```python
from build123d import *

# Parameters (mm, degrees)
CHAMFER1_SIZE = 0.45


with BuildPart() as part:
    # Sketch1 → Revolve1 (revolve)
    with BuildSketch(Plane.XY):
        Polygon((3.25, 0), (3.25, 30.33), (9.44, 30.33), (9.44, 26.03), (11.225, 26.03), (11.225, 24.03), (10.225, 24.03), (10.225, 23.03), (11.225, 23.03), (11.225, 20.53), (12, 20.53), (12, 14.93), (10, 14.93), (10, 12.7), (9.46, 12.7), (9.46, 0), align=None)
    revolve(axis=Axis((0, 0, 0), (0, 1, 0)))

    # Chamfer1
    chamfer1_edges = [part.edges().sort_by_distance(p)[0] for p in [
        (-9.46, 0, 0),
        (-10, 14.93, 0),
        (-3.25, 0, 0),
    ]]
    chamfer(chamfer1_edges, length=CHAMFER1_SIZE)


solid = part.part
```
Here's how the part is built. I have some questions about the finished solid (model axes, mm). A direction names the side the tool comes from. Round coordinates to 2 decimals unless told otherwise and drop trailing zeros. Loops run counter-clockwise (first coordinate to the right, second up) from the corner with the lowest first, then second, coordinate; pieces in that order, holes last.
1. If I drill on probe 1 along X at (y, z) = (23.75, 0) (3 decimals); probe 2 along Z at (x, y) = (0, 13); probe 3 along Y at (x, z) = (-10.5, -2.5), over which ranges is the centre line in solid material (lowest first)?
Answers:
probe 1: x = -10.225 to -3.25, 3.25 to 10.225
probe 2: z = -10 to -3.25, 3.25 to 10
probe 3: y = 14.93 to 23.03, 24.03 to 26.03
2. Suppose I cut it at B-B, the plane y = 24.5. Please give me the cut outline in (x, z) (3 decimals).
Answers:
outline: circle Ø22.45 at (0, 0); hole circle Ø6.5 at (0, 0)
3. Will these pins go through, and if not, where does the flat tip stop? pin 1 (2 mm diameter, centred on x = 5, y = 9.5, fed in from -Z); pin 2 (1 mm diameter, centred on y = 14, z = -2, fed in from +X); pin 3 (1 mm diameter, centred on x = -9.5, z = -7, fed in from -Y).
Answers:
pin 1: stops at z = -8.57
pin 2: stops at x = 9.89
pin 3: stops at y = 14.93
4. Suppose I cut it at A-A, the plane y = 7.5. Please give me the cut outline in (x, z).
Answers:
outline: circle Ø18.92 at (0, 0); hole circle Ø6.5 at (0, 0)
5. For faces 1 (the face through (-11.99, 17.69, -0.53)), 2 (the face through (-10, 23.03, -3)), 3 (the face through (9, 12.7, 4)), 4 (the face through (-8.27, 21.76, -7.59)), 5 (the face through (-4, 30.33, 0)), which set-ups out of +Z, -Z, +X, -X, +Y, -Y let a thin tool reach every point of the face, with its end or its side?
Answers:
face 1: +Y, -Y
face 2: none
face 3: -Y
face 4: +Y
face 5: +Z, -Z, +X, -X, +Y
6. Thinking about a two-plate mould opening in Z: for faces 6 (the face through (-1.23, 6.49, -9.38)), 7 (the face through (-2.579, 15.599, 1.978)), 8 (the face through (-7, 20.53, 9)), which applies, released by +Z, released by -Z, zero draft, split by the parting line, or undercut?
Answers:
face 6: split by the parting line
face 7: undercut
face 8: zero draft
